Autodesk Inventor part; units mm, degrees
ref_plane "YZ Plane" through (0, 0, 0) normal (1, 0, 0) x (0, 1, 0)
ref_plane "XZ Plane" through (0, 0, 0) normal (0, 1, 0) x (-1, 0, 0)
ref_plane "XY Plane" through (0, 0, 0) normal (0, 0, 1) x (1, 0, 0)
sketch "Sketch1" plane through (0, 0, 0) normal (0, 1, 0) x (-1, 0, 0)
  line L0 (0.0752, 55.5625) -> (-25.3248, 55.5625)
  line L1 (-25.3248, 55.5625) -> (-25.3248, -55.5625)
  line L2 (-25.3248, -55.5625) -> (0.0752, -55.5625)
  line L3 (0.0752, -55.5625) -> (0.0752, 55.5625)
  line L4 (54.9786, 0) -> (-47.41, 0) construction
  point P0 (0, 0)
  dimension "d0" = 111.125
  dimension "d1" = 25.4
extrude "Extrusion1" add sketch "Sketch1" along normal blind 120.65
sketch "Sketch2" plane through (25.3248, 0, 55.5625) normal (1, 0, 0) x (0, 0, -1)
  line L0 (55.5625, 0) -> (55.5625, 120.65) construction
  line L1 (0, 120.65) -> (111.125, 120.65) construction
  line L2 (19.05, 120.65) -> (92.075, 120.65)
  line L3 (92.075, 120.65) -> (92.075, 38.1)
  line L4 (92.075, 38.1) -> (19.05, 38.1)
  line L5 (19.05, 38.1) -> (19.05, 120.65)
  line L6 (19.05, 38.1) -> (19.05, 0)
  line L7 (0, 0) -> (111.125, 0)
  line L8 (92.075, 38.1) -> (92.075, 0)
  dimension "d4" = 82.55
  dimension "d10" = 73.025
extrude "Extrusion2" cut sketch "Sketch2" against normal blind 120.65 contours L4 L8 L7 L6
sketch "Sketch3" plane through (25.3248, 0, -55.5625) normal (1, 0, 0) x (0, 0, -1)
  line L0 (-92.075, 38.1) -> (-92.075, 120.65)
  line L1 (-19.05, 120.65) -> (-19.05, 38.1)
  line L2 (0, 0) -> (0, 120.65)
  line L3 (-111.125, 120.65) -> (0, 120.65) construction
  line L4 (-111.125, 0) -> (0, 0)
  line L5 (-111.125, 0) -> (-111.125, 120.65)
  line L6 (-19.05, 38.1) -> (-19.05, 0)
  line L7 (-92.075, 120.65) -> (-19.05, 120.65)
  line L8 (-19.05, 120.65) -> (-19.05, 38.1)
  line L9 (-19.05, 38.1) -> (-92.075, 38.1)
  line L10 (-92.075, 38.1) -> (-92.075, 120.65)
  line L11 (-92.075, 0) -> (-92.075, 38.1)
  line L12 (-111.125, 120.65) -> (-92.075, 120.65)
  line L13 (-92.075, 120.65) -> (-92.075, 0)
  line L14 (-92.075, 0) -> (-111.125, 0)
  line L15 (-111.125, 0) -> (-111.125, 120.65)
  line L16 (-19.05, 120.65) -> (0, 120.65)
  line L17 (0, 120.65) -> (0, 0)
  line L18 (0, 0) -> (-19.05, 0)
  line L19 (-19.05, 0) -> (-19.05, 120.65)
  point P0 (-55.5625, 0)
extrude "Extrusion3" cut sketch "Sketch3" against normal blind 10 contours L11 L4 L5 L12 L0 | L1 L16 L2 L4 L6
sketch "Sketch4" plane through (-0.0752, 0, 55.5625) normal (-1, 0, 0) x (0, 0, 1)
  line L0 (-92.075, 0) -> (-92.075, 38.1)
  line L1 (-92.075, 38.1) -> (-19.05, 38.1)
  line L2 (-19.05, 38.1) -> (-19.05, 0)
  line L3 (-19.05, 0) -> (0, 0)
  line L4 (0, 0) -> (0, 120.65)
  line L5 (-111.125, 120.65) -> (0, 120.65)
  line L6 (-111.125, 0) -> (-111.125, 120.65)
  line L7 (-111.125, 0) -> (-92.075, 0)
  line L8 (-55.5625, 0) -> (-55.5625, 120.65) construction
  line L9 (-111.125, 120.65) -> (0, 120.65) construction
  line L10 (-88.9, 107.95) -> (-22.225, 107.95)
  line L11 (-22.225, 107.95) -> (-22.225, 50.8)
  line L12 (-22.225, 50.8) -> (-88.9, 50.8)
  line L13 (-88.9, 50.8) -> (-88.9, 107.95)
  dimension "d9" = 66.675
  dimension "d11" = 12.7
  dimension "d12" = 12.7
extrude "Extrusion4" cut sketch "Sketch4" against normal blind 23 contours L10 L11 L12 L13
sketch "Sketch5" plane through (25.3248, 38.1, 36.5125) normal (1, 0, 0) x (0, 0, -1)
  line L0 (36.5125, -38.1) -> (36.5125, 82.55) construction
  line L1 (0, 82.55) -> (73.025, 82.55) construction
  line L2 (18.2562, 82.55) -> (54.7687, 82.55)
  line L3 (54.7687, 82.55) -> (54.7687, 53.975)
  line L4 (54.7687, 53.975) -> (18.2562, 53.975)
  line L5 (18.2562, 53.975) -> (18.2562, 82.55)
  circle A0 centre (36.5125, 53.975) radius 18.2563
  dimension "d16" = 36.5125
  dimension "d17" = 28.575
fillet "Fillet1" radius 3.175 4 edges at (11.4248, 107.95, 33.3375) (11.4248, 50.8, 33.3375) (11.4248, 50.8, -33.3375) (11.4248, 107.95, -33.3375)
extrude "Extrusion5" cut sketch "Sketch5" against normal blind 25.4
sketch "Sketch6" plane through (25.3248, 38.1, 36.5125) normal (1, 0, 0) x (0, 0, -1)
  point P0 (36.5125, -38.1)
sketch "Sketch7" plane through (0, 120.65, 0) normal (0, 1, 0) x (1, 0, 0)
  point P0 (0, 0)
  point P1 (6.7165, -47.6926)
properties part number "vertical_face_block" material "Aluminum 6061"
The listing builds one solid part. Answer for the finished solid, in the listing's coordinates (mm). A direction names the side the tool comes from. Round coordinates to 2 decimals unless told otherwise and drop trailing zeros. Loops run counter-clockwise (first coordinate to the right, second up) from the corner with the lowest first, then second, coordinate; pieces in that order, holes last. Notation, with made-up numbers: M -4,46 L 20,46 A11 ccw 20,62 Z; hole C 13.5,16.5 d10. An arc over 180 degrees is marked long. Return JSON: item names as keys, results as strings.
Q1. Find section D-D, the plane y = 63. Determine the outline of the cut face in (x, z).
Results list:
{"outline": "M -0.08,-55.56 L 15.32,-55.56 L 15.32,-36.51 L 25.32,-36.51 L 25.32,36.51 L 15.32,36.51 L 15.32,55.56 L -0.08,55.56 L -0.08,33.34 L 22.92,33.34 L 22.92,-33.34 L -0.08,-33.34 Z"}
Q2. Which of the six approach directions +Z, -Z, +X, -X, +Y, -Y give full straight-line access (tool end or side, diameter ignored) to faces 1 (the face through (13, 113, -18.256)), 2 (the face through (20, 79, 36.512)), 3 (the face through (20, 80, -36.512)), 4 (the face through (11, 50.8, 0))?
Results list:
{"face 1": "+X, -X, +Y", "face 2": "+Z, +X, +Y, -Y", "face 3": "-Z, +X, +Y, -Y", "face 4": "-X"}
Q3. Each of these flat-tipped pins is pushed along its axis until it touches: pin 1 Ø5 at (x, z) = (21, -6.5) entering from +Y; pin 2 Ø5 at (x, y) = (19.5, 59.5) entering from +Z; pin 3 Ø5.5 at (y, z) = (81.5, -49) entering from +X. Where does it stop, or does it pass through?
Results list:
{"pin 1": "stops at y = 75.71", "pin 2": "stops at z = 36.51", "pin 3": "stops at x = 15.32"}
Q4. Find section B-B, the plane y = 10. Determine the outline of the cut face in (x, z), plus the area to 3 significant figures.
Results list:
{"outline": "M -0.08,-55.56 L 15.32,-55.56 L 15.32,-36.51 L -0.08,-36.51 Z; M -0.08,36.51 L 15.32,36.51 L 15.32,55.56 L -0.08,55.56 Z", "area": "587 mm2"}
Q5. Find the intervals of material crossed by line 1 along Y through (x, z) = (2.25, 28.5); line 2 along Z through (x, y) = (21.25, 75); line 3 along Z through (x, y) = (1, 33), in increasing order. Write a range as from..to.
Results list:
{"line 1": "y = 38.1..50.8, 107.95..120.65", "line 2": "z = -36.51..-33.34, 33.34..36.51", "line 3": "z = -55.56..-36.51, 36.51..55.56"}
Q6. Find section C-C, the plane z = -20. Determine the outline of the cut face in (x, y), plus the area to 3 significant figures.
Results list:
{"outline": "M -0.08,38.1 L 25.32,38.1 L 25.32,120.65 L -0.08,120.65 L -0.08,107.95 L 22.92,107.95 L 22.92,50.8 L -0.08,50.8 Z", "area": "782 mm2"}
Q7. The mould has two halves that part along Y. Classify faces 5 (the face through (10, 120.65, -33)), 6 (the face through (11, 79, -33.338)), 7 (the face through (-0.075, 46, -1)), 8 (the face through (13, 38.1, -1)): released by +Y, released by -Y, zero draft, split by the parting line, or undercut.
Results list:
{"face 5": "released by +Y", "face 6": "undercut", "face 7": "zero draft", "face 8": "released by -Y"}
